```python
from build123d import *

# Parameters (mm, degrees)
SKETCH2_W               = 50
SKETCH2_H               = 50
BOSS_EXTRUDE1_DEPTH     = 15
SKETCH3_R               = 11.25
CUT_EXTRUDE1_DEPTH      = 8
SKETCH4_R               = 9
CUT_EXTRUDE2_DEPTH      = 4
SKETCH5_W               = 50
SKETCH5_H               = 50
SKETCH5_R               = 15
CUT_EXTRUDE3_DEPTH      = 12
CUT_EXTRUDE4_DEPTH      = 38.336309405
CUT_EXTRUDE4_DEPTH_BACK = 38.336309405
SKETCH6_R               = 1


with BuildPart() as part:
    # Sketch2 → Boss-Extrude1 (new body)
    with BuildSketch(Plane(origin=(0, 0, 0), x_dir=(1, 0, 0), z_dir=(0, 1, 0))):
        Rectangle(SKETCH2_W, SKETCH2_H)
    extrude(amount=BOSS_EXTRUDE1_DEPTH)

    # Sketch3 → Cut-Extrude1 (cut)
    with BuildSketch(Plane(origin=(0, 15, 0), x_dir=(1, 0, 0), z_dir=(0, 1, 0))):
        with Locations(Location((0, 0, 0), (0, 0, 270))):
            Circle(SKETCH3_R)
    extrude(amount=-CUT_EXTRUDE1_DEPTH, mode=Mode.SUBTRACT)

    # Sketch4 → Cut-Extrude2 (cut)
    with BuildSketch(Plane(origin=(0, 7, 0), x_dir=(1, 0, 0), z_dir=(0, 1, 0))):
        with Locations(Location((0, 0, 0), (0, 0, 270))):
            Circle(SKETCH4_R)
    extrude(amount=-CUT_EXTRUDE2_DEPTH, mode=Mode.SUBTRACT)

    # Sketch5 → Cut-Extrude3 (cut)
    with BuildSketch(Plane(origin=(0, 15, 0), x_dir=(1, 0, 0), z_dir=(0, 1, 0))):
        Rectangle(SKETCH5_W, SKETCH5_H)
        with Locations(Location((0, 0, 0), (0, 0, 270))):
            Circle(SKETCH5_R, mode=Mode.SUBTRACT)
    extrude(amount=-CUT_EXTRUDE3_DEPTH, mode=Mode.SUBTRACT)

    # Sketch6 → Cut-Extrude4 (cut, two sides: drawn at the far end of the back side and taken through both)
    with BuildSketch(Plane(origin=(0, 3, 0), x_dir=(1, 0, 0), z_dir=(0, 1, 0)).offset(-CUT_EXTRUDE4_DEPTH_BACK)):
        with Locations(Location((-19, 19, 0), (0, 0, 270))):
            Circle(SKETCH6_R)
        with Locations(Location((19, 19, 0), (0, 0, 270))):
            Circle(SKETCH6_R)
        with Locations(Location((19, -19, 0), (0, 0, 270))):
            Circle(SKETCH6_R)
        with Locations(Location((-19, -19, 0), (0, 0, 270))):
            Circle(SKETCH6_R)
    extrude(amount=CUT_EXTRUDE4_DEPTH + CUT_EXTRUDE4_DEPTH_BACK, mode=Mode.SUBTRACT)


solid = part.part
```
CAD build for the part. Positions are in the model's coordinates, mm. A direction names the side the tool comes from. Round coordinates to 2 decimals unless told otherwise and drop trailing zeros. Write each loop counter-clockwise with the first axis right and the second up, starting at its lowest first coordinate (ties: lowest second). Pieces come first, ordered by that corner, then holes.
Item 1: Drop flat-ended pins along their axis: pin 1 Ø1.2 at (x, z) = (19, 19) entering from +Y; pin 2 Ø3 at (x, y) = (12.5, 12.5) entering from +Z; pin 3 Ø5 at (y, z) = (12, 2.5) entering from +X; pin 4 Ø2 at (y, z) = (11.5, 6) entering from -X. Give the stop position or say it passes through.
Filled in:
pin 1: passes through
pin 2: stops at z = 10.2
pin 3: stops at x = 15
pin 4: stops at x = -14.14
Item 2: Band-saw the part on D-D on y = 13. Write the cut outline in (x, z).
Filled in:
outline: circle Ø30 at (0, 0); hole circle Ø22.5 at (0, 0)
Item 3: Drill centre lines: L1, parallel to Z at x = -19, y = 1.05; L2, parallel to X at y = 5.4, z = 0. Where is each one in solid material? Low to high.
Filled in:
L1: z = -25 to -20, -18 to 18, 20 to 25
L2: x = -15 to -9, 9 to 15
Item 4: Tool access for faces 1 (the flat face through (0, 0, 0)), 2 (the flat face through (0, 3, 0)): list every direction of +Z, -Z, +X, -X, +Y, -Y with a clear straight run to the whole face (end or side of a thin tool).
Filled in:
face 1: +Z, -Z, +X, -X, -Y
face 2: +Y
Item 5: Mould opens along X. For faces 3 (the flat face through (-25, 1, 0)), 4 (the cylindrical face through (0.66, 9.084, -14.985)), 5 (the cylindrical face through (18, 1, -19)) say: released by +X, released by -X, zero draft, split by the parting line, or undercut.
Filled in:
face 3: released by -X
face 4: split by the parting line
face 5: undercut
Item 6: Band-saw the part on C-C on z = 0. Write the cut outline in (x, y), then the cut area to 3 significant figures.
Filled in:
outline: (-25, 0) - (25, 0) - (25, 3) - (15, 3) - (15, 15) - (11.25, 15) - (11.25, 7) - (9, 7) - (9, 3) - (-9, 3) - (-9, 7) - (-11.25, 7) - (-11.25, 15) - (-15, 15) - (-15, 3) - (-25, 3) - close
area: 258 mm2
Item 7: Band-saw the part on A-A on z = -19. Write the cut outline in (x, y).
Filled in:
outline: (-25, 0) - (-20, 0) - (-20, 3) - (-25, 3) - close; (-18, 0) - (18, 0) - (18, 3) - (-18, 3) - close; (20, 0) - (25, 0) - (25, 3) - (20, 3) - close
Item 8: Band-saw the part on B-B on x = -19. Write the cut outline in (y, z).
Filled in:
outline: (0, -25) - (3, -25) - (3, -20) - (0, -20) - close; (0, -18) - (3, -18) - (3, 18) - (0, 18) - close; (0, 20) - (3, 20) - (3, 25) - (0, 25) - close
